from build123d import *

# Parameters (mm, degrees)
BOSS_EXTRUDE1_DEPTH = 2.54
SHELL1_START        = 6.4516
SHELL1_OUTLINE_W    = 2.3368
SHELL1_OUTLINE_H    = 75.9968
SHELL1_DEPTH        = 368.0968
SHELL1_START_2      = 44.5516
SHELL1_2_OUTLINE_W  = 2.3368
SHELL1_2_OUTLINE_H  = 6.35
SHELL1_2_DEPTH      = 50.5968
SHELL1_START_3      = 165.2016
SHELL1_3_OUTLINE_W  = 2.3368
SHELL1_3_OUTLINE_H  = 6.35
SHELL1_3_DEPTH      = 50.5968
SHELL1_START_4      = 285.8516
SHELL1_4_OUTLINE_W  = 2.3368
SHELL1_4_OUTLINE_H  = 6.35
SHELL1_4_DEPTH      = 50.5968
SHELL1_START_5      = 0.1016
SHELL1_5_OUTLINE_W  = 2.3368
SHELL1_5_OUTLINE_H  = 25.1968
SHELL1_5_DEPTH      = 380.7968


# Read off the part's stored shape, not the designer's step: Shell1
with BuildPart() as part:
    # Sketch1 → Boss-Extrude1 (new body)
    with BuildSketch(Plane(origin=(0, 0, 0), x_dir=(1, 0, 0), z_dir=(0, 1, 0))):
        Polygon((0, 12.434013317), (0, -12.965986683), (6.35, -12.965986683), (6.35, -38.365986683), (44.45, -38.365986683), (44.45, -44.715986683), (95.25, -44.715986683), (95.25, -38.365986683), (165.1, -38.365986683), (165.1, -44.715986683), (215.9, -44.715986683), (215.9, -38.365986683), (285.75, -38.365986683), (285.75, -44.715986683), (336.55, -44.715986683), (336.55, -38.365986683), (374.65, -38.365986683), (374.65, -12.965986683), (381, -12.965986683), (381, 12.434013317), (374.65, 12.434013317), (374.65, 37.834013317), (6.35, 37.834013317), (6.35, 12.434013317), align=None)
    extrude(amount=BOSS_EXTRUDE1_DEPTH)

    # Shell1 outline → Shell1 (cut)
    with BuildSketch(Plane.YZ.offset(SHELL1_START)):
        with Locations((1.27, 0.265986683)):
            Rectangle(SHELL1_OUTLINE_W, SHELL1_OUTLINE_H)
    extrude(amount=SHELL1_DEPTH, mode=Mode.SUBTRACT)

    # Shell1 2 outline → Shell1 2 (cut)
    with BuildSketch(Plane.YZ.offset(SHELL1_START_2)):
        with Locations((1.27, 41.439386683)):
            Rectangle(SHELL1_2_OUTLINE_W, SHELL1_2_OUTLINE_H)
    extrude(amount=SHELL1_2_DEPTH, mode=Mode.SUBTRACT)

    # Shell1 3 outline → Shell1 3 (cut)
    with BuildSketch(Plane.YZ.offset(SHELL1_START_3)):
        with Locations((1.27, 41.439386683)):
            Rectangle(SHELL1_3_OUTLINE_W, SHELL1_3_OUTLINE_H)
    extrude(amount=SHELL1_3_DEPTH, mode=Mode.SUBTRACT)

    # Shell1 4 outline → Shell1 4 (cut)
    with BuildSketch(Plane.YZ.offset(SHELL1_START_4)):
        with Locations((1.27, 41.439386683)):
            Rectangle(SHELL1_4_OUTLINE_W, SHELL1_4_OUTLINE_H)
    extrude(amount=SHELL1_4_DEPTH, mode=Mode.SUBTRACT)

    # Shell1 5 outline → Shell1 5 (cut)
    with BuildSketch(Plane.YZ.offset(SHELL1_START_5)):
        with Locations((1.27, 0.265986683)):
            Rectangle(SHELL1_5_OUTLINE_W, SHELL1_5_OUTLINE_H)
    extrude(amount=SHELL1_5_DEPTH, mode=Mode.SUBTRACT)


solid = part.part
The model under review builds one solid part; all positions refer to its coordinate system, in mm. Give positions to 0.01 mm unless a question says otherwise; leave off trailing zeros. Order: outer loops, then holes, each group sorted by start corner. A loop starts at its lowest first (then second) coordinate and runs counter-clockwise, first axis right, second up. Notation, with made-up numbers: M 36,43.25 L 77,43.25 A21 ccw 77,60.25 Z; hole C 74,27.25 d8. An arc over 180 degrees is marked long. Use one line per item in the form item = value. Start each with the question number.
Item 1: We need section A-A on z = 2.5. Give the boundary of the cut face in (x, y).
Item 2: We need section B-B on x = 304. Give the boundary of the cut face in (y, z).
Item 3: Insertion check: pin 1 Ø1.2 at (y, z) = (2, 41.5) entering from -X; pin 2 Ø0.8 at (y, z) = (1, 27) entering from -X; pin 3 Ø0.8 at (x, y) = (21, 1.5) entering from +Z. Each pin has a flat end and moves straight along its axis. Give the tip position at first contact, or say it passes through.
Completed:
q1.outline = M 0,0 L 381,0 L 381,2.54 L 0,2.54 Z; hole M 0.1,0.1 L 380.9,0.1 L 380.9,2.44 L 0.1,2.44 Z
q2.outline = M 0,-37.83 L 2.54,-37.83 L 2.54,44.72 L 0,44.72 Z; hole M 0.1,-37.73 L 2.44,-37.73 L 2.44,44.61 L 0.1,44.61 Z
q3.pin_1 = 44.45
q3.pin_2 = 6.35
q3.pin_3 = 38.37
